Geometry: final body of the model. Coordinates: model frame, mm. Give positions to 0.01 mm unless a question says otherwise; leave off trailing zeros. Write each loop counter-clockwise with the first axis right and the second up, starting at its lowest first coordinate (ties: lowest second). Pieces come first, ordered by that corner, then holes. Notation, with made-up numbers: M -6,32 L 37,32 A33 cw 37,64 Z; hole C 82.25,68.25 d3. An arc over 180 degrees is marked long. Answer as a JSON object with one key per item and string values.
from build123d import *

# Parameters (mm, degrees)
BOSS_EXTRUDE1_DEPTH      = 2.38125
BOSS_EXTRUDE1_DEPTH_BACK = 2.38125


with BuildPart() as part:
    # Sketch1 → Boss-Extrude1 (new body, two sides)
    with BuildSketch(Plane(origin=(0, 0, 0), x_dir=(1, 0, 0), z_dir=(0, 1, 0))) as boss_extrude1_sk:
        Polygon((0, 0), (0, 22.733), (127, 111.633), (177.8, 111.633), (203.2, 22.733), (203.2, 0), align=None)
    extrude(amount=BOSS_EXTRUDE1_DEPTH)
    extrude(boss_extrude1_sk.sketch, amount=-BOSS_EXTRUDE1_DEPTH_BACK)


solid = part.part
1) Line query: line 1 (Z direction, x = 107, y = -1.2); line 2 (X direction, y = -0.3, z = -88.5); line 3 (Z direction, x = 30.5, y = -1.15). Output: solid intervals per line, ascending. Write a range as from..to.
Geometry check:
{"line 1": "z = -97.63..0", "line 2": "x = 93.95..184.41", "line 3": "z = -44.08..0"}
2) Cut plane B-B on x = 17. Return loops of the section in (y, z), and give its area (3 significant figures).
Geometry check:
{"outline": "M -2.38,-34.63 L 2.38,-34.63 L 2.38,0 L -2.38,0 Z", "area": "165 mm2"}
3) Cut plane C-C on z = -99. Return loops of the section in (x, y).
Geometry check:
{"outline": "M 108.95,-2.38 L 181.41,-2.38 L 181.41,2.38 L 108.95,2.38 Z"}
4) Cut plane A-A on y = 1.3. Return loops of the section in (x, z).
Geometry check:
{"outline": "M 0,-22.73 L 127,-111.63 L 177.8,-111.63 L 203.2,-22.73 L 203.2,0 L 0,0 Z"}
